```python
from build123d import *

# Parameters (mm, degrees)
F0_W     = 22.86
F0_H     = 83.82
F1_DEPTH = 22.86
F3_DEPTH = 19.05
F5_DEPTH = 7.62
F6_W     = 6.35
F6_H     = 6.35
F7_DEPTH = 7.62
F9_DEPTH = 7.62


with BuildPart() as f1:
    # F0 (on Top) → F1 (new body)
    with BuildSketch(Plane.XY):
        with Locations((11.43, 41.91)):
            Rectangle(F0_W, F0_H)
    extrude(amount=F1_DEPTH)

    # F2 (on face) → F3 (join)
    with BuildSketch(Plane(origin=(0, 83.82, 0), x_dir=(-1, 0, 0), z_dir=(0, 1, 0))):
        Polygon((-8.255, 8.255), (-8.255, 14.605), (-14.605, 14.605), (-14.605, 11.43), (-14.605, 8.255), align=None)
    extrude(amount=F3_DEPTH)

    # F4 (on face) → F5 (join)
    with BuildSketch(Plane.XZ):
        Polygon((20.32, 20.559318), (2.54, 20.559318), (2.54, 11.43), (2.54, 2.300682), (20.32, 2.300682), align=None)
    extrude(amount=F5_DEPTH)

    # F6 (on face) → F7 (join)
    with BuildSketch(Plane.XZ.offset(7.62)):
        with Locations((8.255, 14.605)):
            Rectangle(F6_W, F6_H)
        Polygon((11.43, 11.43), (5.08, 11.43), (5.08, 5.08), (17.78, 5.08), (17.78, 17.78), (11.43, 17.78), align=None)
    extrude(amount=F7_DEPTH)

    # F8 (on face) → F9 (join)
    with BuildSketch(Plane.XZ.offset(15.24)):
        Polygon((14.605, 15.194485), (8.255, 15.194485), (8.255, 11.43), (8.255, 7.665515), (14.605, 7.665515), align=None)
    extrude(amount=F9_DEPTH)


solid = f1.part
```
The model under review builds one solid part; all positions refer to its coordinate system, in mm. A direction names the side the tool comes from. Round coordinates to 2 decimals unless told otherwise and drop trailing zeros. Write each loop counter-clockwise with the first axis right and the second up, starting at its lowest first coordinate (ties: lowest second). Pieces come first, ordered by that corner, then holes. Notation, with made-up numbers: (-13.75, 63) -> (-8.75, 63) arc R5 ccw to (-8.75, 70) -> close; hole circle Ø4 at (-37.75, 69.5). An arc over 180 degrees is marked (long way). Use CSV: the item, a comma, the result in double quotes.
Q1. For pin 1 Ø4 at (y, z) = (-19.5, 10.5) entering from -X (3 decimals); pin 2 Ø7 at (x, y) = (11, 89) entering from +Z (3 decimals); pin 3 Ø4 at (y, z) = (-4, 15) entering from -X, all flat-tipped, find the tip position at first contact; note any pin that passes through.
Checks:
pin 1,"x = 8.255"
pin 2,"z = 14.605"
pin 3,"x = 2.54"
Q2. For faces 1 (the flat face through (20.32, -4, 11)), 2 (the flat face through (11, 93, 8.255)), 3 (the flat face through (12, -11, 17.78)), list the 3-axis set-ups (+Z, -Z, +X, -X, +Y, -Y) from which the entire face can be reached by the end or side of a thin tool; tool diameter is ignored.
Checks:
face 1,"+Z, -Z, +X, -Y"
face 2,"-Z, +X, -X, +Y"
face 3,"+Z, +X, -X, -Y"
Q3. Consider section D-D (z = 12.5). Give the boundary of the cut face in (x, y) (3 decimals).
Checks:
outline,"(0, 0) -> (2.54, 0) -> (2.54, -7.62) -> (5.08, -7.62) -> (5.08, -15.24) -> (8.255, -15.24) -> (8.255, -22.86) -> (14.605, -22.86) -> (14.605, -15.24) -> (17.78, -15.24) -> (17.78, -7.62) -> (20.32, -7.62) -> (20.32, 0) -> (22.86, 0) -> (22.86, 83.82) -> (14.605, 83.82) -> (14.605, 102.87) -> (8.255, 102.87) -> (8.255, 83.82) -> (0, 83.82) -> close"
Q4. To check wall thickness, follow probe 1 along Z at (x, y) = (10.5, -4); probe 2 along Z at (x, y) = (7, -13.5); probe 3 along Y at (x, z) = (21.25, 17.5). State the ranges of each line that lie inside material, in increasing order. Write a range as [from, to].
Checks:
probe 1,"[2.3, 20.56]"
probe 2,"[5.08, 17.78]"
probe 3,"[0, 83.82]"
Q5. Consider section B-B (x = 11). Give the boundary of the cut face in (y, z) (3 decimals).
Checks:
outline,"(-22.86, 7.666) -> (-15.24, 7.666) -> (-15.24, 5.08) -> (-7.62, 5.08) -> (-7.62, 2.301) -> (0, 2.301) -> (0, 0) -> (83.82, 0) -> (83.82, 8.255) -> (102.87, 8.255) -> (102.87, 14.605) -> (83.82, 14.605) -> (83.82, 22.86) -> (0, 22.86) -> (0, 20.559) -> (-7.62, 20.559) -> (-7.62, 17.78) -> (-15.24, 17.78) -> (-15.24, 15.194) -> (-22.86, 15.194) -> close"
Q6. Consider section C-C (y = -10). Give the boundary of the cut face in (x, z).
Checks:
outline,"(5.08, 5.08) -> (17.78, 5.08) -> (17.78, 17.78) -> (5.08, 17.78) -> close"
Q7. Consider section A-A (z = 6.5). Give the boundary of the cut face in (x, y), then the cut area to 3 significant figures.
Checks:
outline,"(0, 0) -> (2.54, 0) -> (2.54, -7.62) -> (5.08, -7.62) -> (5.08, -15.24) -> (17.78, -15.24) -> (17.78, -7.62) -> (20.32, -7.62) -> (20.32, 0) -> (22.86, 0) -> (22.86, 83.82) -> (0, 83.82) -> close"
area,"2,150 mm²"
